```python
from build123d import *

# Parameters (mm, degrees)
SKETCH1_R           = 28
SKETCH1_R_2         = 15
BOSS_EXTRUDE1_DEPTH = 34
SKETCH2_R           = 1.5
CUT_EXTRUDE1_DEPTH  = 4
CIRPATTERN1_COUNT   = 2


with BuildPart() as part:
    # Sketch1 → Boss-Extrude1 (new body)
    with BuildSketch(Plane.XY):
        Circle(SKETCH1_R)
        Circle(SKETCH1_R_2, mode=Mode.SUBTRACT)
    extrude(amount=-BOSS_EXTRUDE1_DEPTH)

    # Sketch2 → Cut-Extrude1 (cut)
    with BuildSketch(Plane(origin=(0, 0, -34), x_dir=(-1, 0, 0), z_dir=(0, 0, -1))):
        with Locations((3, 23)):
            Circle(SKETCH2_R)
        with Locations((-3, 23)):
            Circle(SKETCH2_R)
    cut_extrude1 = extrude(amount=-CUT_EXTRUDE1_DEPTH, mode=Mode.SUBTRACT)

    # CirPattern1: Cut-Extrude1 ×2 about axis
    cirpattern1_axis = Axis((0, 0, 0), (0, 0, 1))
    for i in range(1, CIRPATTERN1_COUNT):
        add(cut_extrude1.rotate(cirpattern1_axis, i * 360 / CIRPATTERN1_COUNT), mode=Mode.SUBTRACT)


solid = part.part
```
Design review of the part built by this model. Coordinates are the model's own, in mm. A direction names the side the tool comes from. Give positions to 0.01 mm unless a question says otherwise; leave off trailing zeros. Loops run counter-clockwise (first coordinate to the right, second up) from the corner with the lowest first, then second, coordinate; pieces in that order, holes last. Notation, with made-up numbers: M -9.75,14.5 L 33.25,14.5 A25 cw 33.25,30.5 Z; hole C 1,66.5 d6. An arc over 180 degrees is marked long. Return JSON: item names as keys, results as strings. Group by question number.
Item 1: We need section D-D (y = -23). Give the boundary of the cut face in (x, z), and give its area (3 significant figures).
Item 2: Mouldability with a two-part tool opening along X and no side actions: class faces 3 (the cylindrical face through (2.805, -24.487, -32.028)), 4 (the flat face through (12, -12, 0)), 5 (the cylindrical face through (25.865, -10.724, -16.762)), 6 (the cylindrical face through (-14.985, 0.66, -16.762)) as released by +X, released by -X, zero draft, split by the parting line, or undercut.
Item 3: Insertion check: pin 1 Ø3 at (x, z) = (-4, -30) entering from -Y; pin 2 Ø12 at (x, z) = (12.5, -22) entering from -Y; pin 3 Ø3 at (x, z) = (-14, -11.5) entering from +Y. Each pin has a flat end and moves straight along its axis. Give the tip position at first contact, or say it passes through.
Item 4: Tool access review of faces 1 (the flat face through (-3, 23, -30)), 2 (the flat face through (12, -12, -34)): name each direction out of +Z, -Z, +X, -X, +Y, -Y from which nothing blocks a thin tool from reaching the whole face with its end or side.
Item 5: We need section C-C (z = -23). Give the boundary of the cut face in (x, y), and give its area (3 significant figures).
Item 6: We need section A-A (x = 0). Give the boundary of the cut face in (y, z), and give its area (3 significant figures).
Item 7: For probe 1 along Y at (x, z) = (-3, -30.9); probe 2 along X at (y, z) = (-23, -32); probe 3 along X at (y, z) = (2, -6), list the stretches that pass through material, from the lowest coordinate up.
Output:
{
 "1": {"outline": "M -15.97,-34 L -4.5,-34 L -4.5,-30 L -1.5,-30 L -1.5,-34 L 1.5,-34 L 1.5,-30 L 4.5,-30 L 4.5,-34 L 15.97,-34 L 15.97,0 L -15.97,0 Z", "area": "1,060 mm^2"},
 "2": {"face 3": "undercut", "face 4": "zero draft", "face 5": "split by the parting line", "face 6": "undercut"},
 "3": {"pin 1": "stops at y = -27.89", "pin 2": "stops at y = -27.24", "pin 3": "stops at y = 25.05"},
 "4": {"face 1": "-Z", "face 2": "-Z, +X, -X, +Y, -Y"},
 "5": {"outline": "C 0,0 d56; hole C 0,0 d30", "area": "1,760 mm^2"},
 "6": {"outline": "M -28,-34 L -15,-34 L -15,0 L -28,0 Z; M 15,-34 L 28,-34 L 28,0 L 15,0 Z", "area": "884 mm^2"},
 "7": {"probe 1": "y = -27.84 to -24.5, -21.5 to -14.7, 14.7 to 21.5, 24.5 to 27.84", "probe 2": "x = -15.97 to -4.5, -1.5 to 1.5, 4.5 to 15.97", "probe 3": "x = -27.93 to -14.87, 14.87 to 27.93"}
}
